The listing builds one solid part. Answer for the finished solid, in the listing's coordinates (mm). Face numbers are marked on the shaded views. A direction names the side the tool comes from. Give positions to 0.01 mm unless a question says otherwise; leave off trailing zeros. Write each loop counter-clockwise with the first axis right and the second up, starting at its lowest first coordinate (ties: lowest second). Pieces come first, ordered by that corner, then holes. Notation, with made-up numbers: (-37, 26) -> (10, 26) arc R13 cw to (10, 40) -> close; hole circle Ø11 at (68.25, 62). An arc over 180 degrees is marked (long way). Put each result on its own line as item: value. Start each with the question number.
1) A cutting plane is placed at B-B (z = 85). Write down the section's boundary in (x, y).
2) A cutting plane is placed at C-C (x = -86.5). Write down the section's boundary in (y, z).
3) Flat-ended cylindrical pins translate along their axes: pin 1 Ø8 at (x, y) = (-78.5, -19) entering from -Z; pin 2 Ø6 at (y, z) = (-18, 92.5) entering from -X; pin 3 Ø22 at (x, z) = (-90.5, 89) entering from -Y. Find the tip coordinate at first contact, or state that the pin passes through.
4) A cutting plane is placed at D-D (y = -14). Write down the section's boundary in (x, z).
5) Find the intervals of material crossed by line 1 along Y through (x, z) = (-27.5, 35); line 2 along Z through (x, y) = (-70.5, -16) (3 decimals); line 3 along Z through (x, y) = (-33, -7), in increasing order. Write a range as from..to.
6) For the marked faces 4 and 5, determine the directions among +Z, -Z, +X, -X, +Y, -Y from which every point of the face is accessible in a straight line to the end or side of a thin tool.
7) A cutting plane is placed at A-A (y = -22). Write down the section's boundary in (x, z).
8) For a pull along X with two mould halves and no side action, classify the marked faces 1, 2 and 3 as released by +X, released by -X, zero draft, split by the parting line, or undercut.
from build123d import *

# Parameters (mm, degrees)
F0_R     = 9
F0_R_2   = 10
F1_DEPTH = 32
F2_R     = 10
F3_DEPTH = 15
F4_W     = 48
F4_H     = 16
F5_DEPTH = 105.001


with BuildPart() as f1:
    # F0 (on Front) → F1 (new body)
    with BuildSketch(Plane.XZ):
        with BuildLine():
            Line((-70, 0), (0, 0))
            Line((0, 0), (0, 12))
            Line((0, 12), (-30, 12))
            ThreePointArc((-30, 12), (-38, 20), (-30, 28))
            Line((-30, 28), (0, 28))
            Line((0, 28), (0, 40))
            ThreePointArc((0, 40), (-32.741064, 51.374572), (-58.1024, 75))
            Line((-58.1024, 75), (-64.259527, 75))
            ThreePointArc((-64.259527, 75), (-82.050541, 61.34016), (-103.358452, 68.346179))
            Line((-103.358452, 68.346179), (-94.590621, 20.494296))
            ThreePointArc((-94.590621, 20.494296), (-86.005584, 5.795279), (-70, 0))
        make_face()
        with Locations((-70, 25)):
            Circle(F0_R, mode=Mode.SUBTRACT)
        with BuildLine():
            Line((-105.749448, 81.395437), (-103.358452, 68.346179))
            ThreePointArc((-103.358452, 68.346179), (-82.050541, 61.34016), (-64.259527, 75))
            Line((-64.259527, 75), (-58.1024, 75))
            ThreePointArc((-58.1024, 75), (-63.305667, 83.4088), (-67.484714, 92.370801))
            ThreePointArc((-67.484714, 92.370801), (-91.591151, 104.224817), (-105.749448, 81.395437))
        make_face()
        with Locations((-86.076952, 85)):
            Circle(F0_R_2, mode=Mode.SUBTRACT)
    extrude(amount=F1_DEPTH)

    # F2 (on face) → F3 (cut)
    with BuildSketch(Plane.XZ.offset(32)):
        with BuildLine():
            ThreePointArc((-67.484714, 92.370801), (-91.591151, 104.224817), (-105.749448, 81.395437))
            Line((-105.749448, 81.395437), (-103.358452, 68.346179))
            ThreePointArc((-103.358452, 68.346179), (-82.050541, 61.34016), (-64.259527, 75))
            Line((-64.259527, 75), (-58.1024, 75))
            ThreePointArc((-58.1024, 75), (-63.305667, 83.4088), (-67.484714, 92.370801))
        make_face()
        with Locations((-86.076952, 85)):
            Circle(F2_R, mode=Mode.SUBTRACT)
    extrude(amount=-F3_DEPTH, mode=Mode.SUBTRACT)

    # F4 (on face) → F5 (cut, through all)
    with BuildSketch(Plane(origin=(0, 0, 0), x_dir=(1, 0, 0), z_dir=(0, 0, -1))):
        with Locations((-24, 16)):
            Rectangle(F4_W, F4_H)
    extrude(amount=-F5_DEPTH, mode=Mode.SUBTRACT)


solid = f1.part
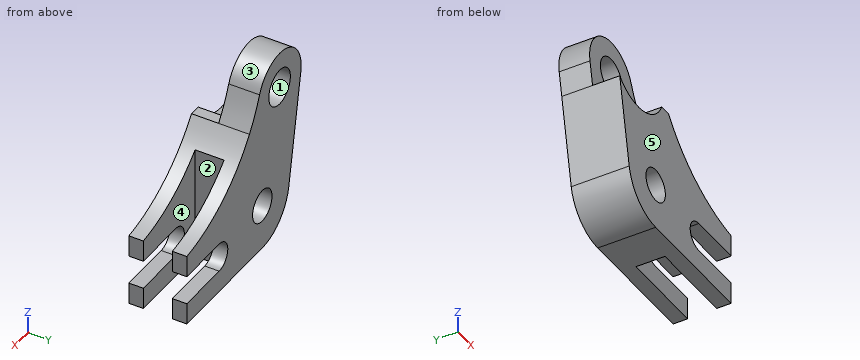
Reply:
1. outline: (-106.08, -17) -> (-96.08, -17) -> (-96.08, 0) -> (-106.08, 0) -> close; (-76.08, -17) -> (-64.14, -17) -> (-64.14, 0) -> (-76.08, 0) -> close
2. outline: (-32, 6.22) -> (0, 6.22) -> (0, 75.01) -> (-17, 75.01) -> (-17, 61) -> (-32, 61) -> close; (-17, 94.99) -> (0, 94.99) -> (0, 105) -> (-17, 105) -> close
3. pin 1: stops at z = 0.41
3. pin 2: stops at x = -105.52
3. pin 3: stops at y = -17
4. outline: (-105.75, 81.4) -> (-94.59, 20.49) arc R25 ccw to (-70, 0) -> (-48, 0) -> (-48, 63.15) arc R84 cw to (-58.1, 75) arc R84 cw to (-67.48, 92.37) arc R20 ccw to start; hole circle Ø20 at (-86.08, 85); hole circle Ø18 at (-70, 25)
5. line 1: y = -32..-24, -8..0
5. line 2: z = 0.005..16.014, 33.986..97.544
5. line 3: z = 0..12.58, 27.42..51.53
6. face 4: +Z, -Z, +X
6. face 5: +Z, -Z, +X, -X, -Y
7. outline: (-103.36, 68.35) -> (-94.59, 20.49) arc R25 ccw to (-70, 0) -> (-48, 0) -> (-48, 63.15) arc R84 cw to (-58.1, 75) -> (-64.26, 75) arc R24 cw to start; hole circle Ø18 at (-70, 25)
8. face 1: undercut
8. face 2: released by +X
8. face 3: split by the parting line
